from build123d import *

# Parameters (mm, degrees)
BOSS_EXTRU_1_DEPTH = 320


with BuildPart() as part:
    # Esquisse1 → Boss.-Extru.1 (new body)
    with BuildSketch(Plane.XY):
        with BuildLine():
            Line((-9.5, 10), (-4.58, 10))
            Line((-4.58, 10), (-3.125, 8.545))
            Line((-3.125, 8.545), (-3.125, 8.2))
            Line((-3.125, 8.2), (-5.5, 8.2))
            Line((-5.5, 8.2), (-5.5, 6.560660172))
            Line((-5.5, 6.560660172), (-2.839339828, 3.9))
            Line((-2.839339828, 3.9), (-0.21, 3.9))
            Line((-0.21, 3.9), (0, 3.69))
            Line((0, 3.69), (0, 2.1))
            ThreePointArc((0, 2.1), (-2.1, 0), (0, -2.1))
            Line((0, -2.1), (0, -3.69))
            Line((0, -3.69), (-0.21, -3.9))
            Line((-0.21, -3.9), (-2.839339828, -3.9))
            Line((-2.839339828, -3.9), (-6.239339828, -7.3))
            Line((-6.239339828, -7.3), (-8.2, -7.3))
            Line((-8.2, -7.3), (-8.2, -12.7))
            Line((-8.2, -12.7), (-6.239339828, -12.7))
            Line((-6.239339828, -12.7), (-2.839339828, -16.1))
            Line((-2.839339828, -16.1), (-0.21, -16.1))
            Line((-0.21, -16.1), (0, -16.31))
            Line((0, -16.31), (0, -17.9))
            ThreePointArc((0, -17.9), (-2.1, -20), (0, -22.1))
            Line((0, -22.1), (0, -23.69))
            Line((0, -23.69), (-0.21, -23.9))
            Line((-0.21, -23.9), (-2.839339828, -23.9))
            Line((-2.839339828, -23.9), (-6.239339828, -27.3))
            Line((-6.239339828, -27.3), (-8.2, -27.3))
            Line((-8.2, -27.3), (-8.2, -32.7))
            Line((-8.2, -32.7), (-6.239339828, -32.7))
            Line((-6.239339828, -32.7), (-2.839339828, -36.1))
            Line((-2.839339828, -36.1), (-0.21, -36.1))
            Line((-0.21, -36.1), (0, -36.31))
            Line((0, -36.31), (0, -37.9))
            ThreePointArc((0, -37.9), (-2.1, -40), (0, -42.1))
            Line((0, -42.1), (0, -43.69))
            Line((0, -43.69), (-0.21, -43.9))
            Line((-0.21, -43.9), (-2.839339828, -43.9))
            Line((-2.839339828, -43.9), (-5.5, -46.560660172))
            Line((-5.5, -46.560660172), (-5.5, -48.2))
            Line((-5.5, -48.2), (-3.125, -48.2))
            Line((-3.125, -48.2), (-3.125, -48.545))
            Line((-3.125, -48.545), (-4.58, -50))
            Line((-4.58, -50), (-9.5, -50))
            ThreePointArc((-9.5, -50), (-9.853553391, -49.853553391), (-10, -49.5))
            Line((-10, -49.5), (-10, -44.58))
            Line((-10, -44.58), (-8.545, -43.125))
            Line((-8.545, -43.125), (-8.2, -43.125))
            Line((-8.2, -43.125), (-8.2, -45.5))
            Line((-8.2, -45.5), (-6.560660172, -45.5))
            Line((-6.560660172, -45.5), (-3.9, -42.839339828))
            Line((-3.9, -42.839339828), (-3.9, -40.21))
            Line((-3.9, -40.21), (-3.69, -40))
            Line((-3.69, -40), (-3.9, -39.79))
            Line((-3.9, -39.79), (-3.9, -37.160660172))
            Line((-3.9, -37.160660172), (-6.560660172, -34.5))
            Line((-6.560660172, -34.5), (-8.2, -34.5))
            Line((-8.2, -34.5), (-8.2, -36.875))
            Line((-8.2, -36.875), (-8.545, -36.875))
            Line((-8.545, -36.875), (-10, -35.42))
            Line((-10, -35.42), (-10, -24.58))
            Line((-10, -24.58), (-8.545, -23.125))
            Line((-8.545, -23.125), (-8.2, -23.125))
            Line((-8.2, -23.125), (-8.2, -25.5))
            Line((-8.2, -25.5), (-6.560660172, -25.5))
            Line((-6.560660172, -25.5), (-3.9, -22.839339828))
            Line((-3.9, -22.839339828), (-3.9, -20.21))
            Line((-3.9, -20.21), (-3.69, -20))
            Line((-3.69, -20), (-3.9, -19.79))
            Line((-3.9, -19.79), (-3.9, -17.160660172))
            Line((-3.9, -17.160660172), (-6.560660172, -14.5))
            Line((-6.560660172, -14.5), (-8.2, -14.5))
            Line((-8.2, -14.5), (-8.2, -16.875))
            Line((-8.2, -16.875), (-8.545, -16.875))
            Line((-8.545, -16.875), (-10, -15.42))
            Line((-10, -15.42), (-10, -4.58))
            Line((-10, -4.58), (-8.545, -3.125))
            Line((-8.545, -3.125), (-8.2, -3.125))
            Line((-8.2, -3.125), (-8.2, -5.5))
            Line((-8.2, -5.5), (-6.560660172, -5.5))
            Line((-6.560660172, -5.5), (-3.9, -2.839339828))
            Line((-3.9, -2.839339828), (-3.9, -0.21))
            Line((-3.9, -0.21), (-3.69, 0))
            Line((-3.69, 0), (-3.9, 0.21))
            Line((-3.9, 0.21), (-3.9, 2.839339828))
            Line((-3.9, 2.839339828), (-6.560660172, 5.5))
            Line((-6.560660172, 5.5), (-8.2, 5.5))
            Line((-8.2, 5.5), (-8.2, 3.125))
            Line((-8.2, 3.125), (-8.545, 3.125))
            Line((-8.545, 3.125), (-10, 4.58))
            Line((-10, 4.58), (-10, 9.5))
            ThreePointArc((-10, 9.5), (-9.853553391, 9.853553391), (-9.5, 10))
        make_face()
    boss_extru_1 = extrude(amount=BOSS_EXTRU_1_DEPTH)

    # Symétrie1: Boss.-Extru.1 across plane
    add(boss_extru_1.mirror(Plane(origin=(0, 3.69, 320), x_dir=(0, 0, 1), z_dir=(-1, 0, 0))))


solid = part.part
Design review of the part built by this model. Coordinates are the model's own, in mm. A direction names the side the tool comes from. Give positions to 0.01 mm unless a question says otherwise; leave off trailing zeros. Return JSON: item names as keys, results as strings. Group by question number.
Item 1: Take a section at A-A (z = 198). Count the separate pieces of the cut face and the enclosed holes in it, plus the area to 3 significant figures.
Item 2: Clearance check with flat-ended pins moving along their axes: pin 1 Ø0.7 at (y, z) = (-24, 233) entering from -X; pin 2 Ø2 at (x, z) = (3, 139.5) entering from -Y; pin 3 Ø2 at (y, z) = (-22, 162.5) entering from +X. State where each tip first meets the part, or that it passes through.
Item 3: The part is to be moulded in two halves that separate along X. For faces 3 (the flat face through (-2.4, -19.6, 320)), 4 (the flat face through (-10, -47, 158)), 5 (the flat face through (-8.2, -30, 158)), say which applies: pulls with the +X half, pulls with the -X half, needs draft (parallel to the pull), parting line crosses it, or undercut.
Item 4: Wall thickness on line 1 along Y through (x, z) = (2.5, 210); line 2 along Y through (x, z) = (-8.25, 158) (3 decimals); line 3 along Y through (x, z) = (-7, 303): over which ranges is each line inside the solid? List them lowest first.
Item 5: Tool access review of faces 1 (the flat face through (10, -30, 158)), 2 (the flat face through (-8.2, -10, 158)): name each direction out of +Z, -Z, +X, -X, +Y, -Y from which nothing blocks a thin tool from reaching the whole face with its end or side.
Return value:
{
 "1": {"separate pieces": "1", "enclosed holes": "5", "area": "428 mm2"},
 "2": {"pin 1": "stops at x = -9.77", "pin 2": "stops at y = -49.42", "pin 3": "stops at x = 4.06"},
 "3": {"face 3": "needs draft", "face 4": "pulls with the -X half", "face 5": "undercut"},
 "4": {"line 1": "y = -43.9 to -36.1, -23.9 to -16.1, -3.9 to 3.9", "line 2": "y = -50 to -43.125, -36.875 to -23.125, -16.875 to -3.125, 3.125 to 10", "line 3": "y = -50 to -45.5, -34.5 to -32.7, -27.3 to -25.5, -14.5 to -12.7, -7.3 to -5.5, 5.5 to 10"},
 "5": {"face 1": "+Z, -Z, +X, +Y, -Y", "face 2": "+Z, -Z"}
}
